Can you work these out from the model? Positions are in its coordinate system, mm. A direction names the side the tool comes from. Round coordinates to 2 decimals unless told otherwise and drop trailing zeros. Loops run counter-clockwise (first coordinate to the right, second up) from the corner with the lowest first, then second, coordinate; pieces in that order, holes last. Notation, with made-up numbers: M 65.25,-13 L 120.25,-13 A15 ccw 120.25,6 Z; hole C 86,50.25 d6. An arc over 180 degrees is marked long. Answer as CSV lines item,"result".
from build123d import *

# Parameters (mm, degrees)
SKETCH_1_W      = 74
SKETCH_1_H      = 25
SKETCH_1_R      = 1.5
EXTRUDE_1_DEPTH = 2
SKETCH_2_R      = 5
SKETCH_2_R_2    = 1.5
EXTRUDE_2_DEPTH = 2


with BuildPart() as part:
    # Эскиз1 → Бобышка-Вытянуть1 (new body)
    with BuildSketch(Plane(origin=(0, 0, 0), x_dir=(1, 0, 0), z_dir=(0, 1, 0))):
        with Locations((37, 12.5)):
            Rectangle(SKETCH_1_W, SKETCH_1_H)
        with Locations((7, 18)):
            Circle(SKETCH_1_R, mode=Mode.SUBTRACT)
        with Locations((67, 18)):
            Circle(SKETCH_1_R, mode=Mode.SUBTRACT)
        with Locations((7, 7)):
            Circle(SKETCH_1_R, mode=Mode.SUBTRACT)
        with Locations((67, 7)):
            Circle(SKETCH_1_R, mode=Mode.SUBTRACT)
    extrude(amount=EXTRUDE_1_DEPTH)

    # Эскиз2 → Бобышка-Вытянуть2 (add)
    with BuildSketch(Plane.XY):
        with BuildLine():
            Line((0, 2), (74, 2))
            Line((74, 2), (74, -21))
            ThreePointArc((74, -21), (67.556349186, -36.556349186), (52, -43))
            Line((52, -43), (22, -43))
            ThreePointArc((22, -43), (6.443650814, -36.556349186), (0, -21))
            Line((0, -21), (0, 2))
        make_face()
        with Locations((37, -28.5)):
            Circle(SKETCH_2_R, mode=Mode.SUBTRACT)
        with Locations((28.354168617, -13.306972233)):
            Circle(SKETCH_2_R_2, mode=Mode.SUBTRACT)
        with Locations((48.525028222, -21.173764644)):
            Circle(SKETCH_2_R_2, mode=Mode.SUBTRACT)
        with Locations((31.626756345, -34.708845272)):
            Circle(SKETCH_2_R_2, mode=Mode.SUBTRACT)
    extrude(amount=-EXTRUDE_2_DEPTH)


solid = part.part
Item 1: Will these pins go through, and if not, where does the flat tip stop? pin 1 (3.5 mm diameter, centred on x = 67, z = -18, fed in from -Y); pin 2 (13 mm diameter, centred on x = 27, y = -22, fed in from -Z).
Output:
pin 1,"stops at y = 0"
pin 2,"stops at z = -2"
Item 2: If we section it at C-C on x = 67.5: Write out the boundary of the cut face in (y, z).
Output:
outline,"M -36.61,-2 L 0,-2 L 0,-5.59 L 2,-5.59 L 2,0 L -36.61,0 Z; M 0,-25 L 2,-25 L 2,-19.41 L 0,-19.41 Z; M 0,-16.59 L 2,-16.59 L 2,-8.41 L 0,-8.41 Z"
Item 3: If we section it at A-A on z = -18: Write out the boundary of the cut face in (x, y).
Output:
outline,"M 0,0 L 5.5,0 L 5.5,2 L 0,2 Z; M 8.5,0 L 65.5,0 L 65.5,2 L 8.5,2 Z; M 68.5,0 L 74,0 L 74,2 L 68.5,2 Z"
Item 4: If I drill on line 1 along X through (y, z) = (1.25, -18); line 2 along Y through (x, z) = (56, -17.5); line 3 along Z through (x, y) = (68, -14.5), over which ranges is the centre line in solid material (lowest first)? Write a range as from..to.
Output:
line 1,"x = 0..5.5, 8.5..65.5, 68.5..74"
line 2,"y = 0..2"
line 3,"z = -2..0"
Item 5: If we section it at B-B on x = 37: Write out the boundary of the cut face in (y, z), then the cut area to 3 significant figures.
Output:
outline,"M -43,-2 L -33.5,-2 L -33.5,0 L -43,0 Z; M -23.5,-2 L 0,-2 L 0,-25 L 2,-25 L 2,0 L -23.5,0 Z"
area,"116 mm2"
Item 6: We'd pull the mould along X, two halves only. Please class faces 3 (the face through (36, -21, 0)), 4 (the face through (26.856, -13.241, -0.986)), 5 (the face through (74, 1, -7)), 6 (the face through (32.32, -36.04, -0.99)): released by +X, released by -X, zero draft, split by the parting line, or undercut.
Output:
face 3,"zero draft"
face 4,"undercut"
face 5,"released by +X"
face 6,"undercut"
Item 7: On a 3-axis mill with a long thin cutter (end or side, diameter ignored), from which of +Z, -Z, +X, -X, +Y, -Y can I reach the whole of each face in a straight line? I mean faces 1 (the face through (36, 0, -14)), 2 (the face through (6.62, -36.73, -0.99)). Say none if no direction works.
Output:
face 1,"-Z, +X, -X, -Y"
face 2,"+Z, -Z, -X, -Y"
Item 8: If we section it at D-D on y = -28.5: Write out the boundary of the cut face in (x, z).
Output:
outline,"M 1.32,-2 L 32,-2 L 32,0 L 1.32,0 Z; M 42,-2 L 72.68,-2 L 72.68,0 L 42,0 Z"
